Source: CAD feature listing. Evaluate the final solid. Frame: model axes, mm. A direction names the side the tool comes from. Round coordinates to 2 decimals unless told otherwise and drop trailing zeros. Write each loop counter-clockwise with the first axis right and the second up, starting at its lowest first coordinate (ties: lowest second). Pieces come first, ordered by that corner, then holes.
```python
from build123d import *

# Parameters (mm, degrees)
BOSS_EXTRUDE1_DEPTH = 3
SKETCH2_R           = 2.1
CUT_EXTRUDE1_DEPTH  = 3
BOSS_EXTRUDE2_DEPTH = 27
CUT_EXTRUDE2_DEPTH  = 27
RIB1_REACH          = 75.171
SKETCH5_WALL_W      = 155.413132852
SKETCH5_WALL_H      = 1
RIB2_REACH          = 75.171
SKETCH6_WALL_W      = 155.413132852
SKETCH6_WALL_H      = 1


with BuildPart() as part:
    # Sketch1 → Boss-Extrude1 (new body)
    with BuildSketch(Plane(origin=(0, 0, 0), x_dir=(1, 0, 0), z_dir=(0, 1, 0))):
        Polygon((0, 0), (0, 23), (12, 23), (12, 3), (52, 3), (52, 23), (64, 23), (64, 0), align=None)
    extrude(amount=-BOSS_EXTRUDE1_DEPTH)

    # Sketch2 → Cut-Extrude1 (cut)
    with BuildSketch(Plane(origin=(0, -3, 0), x_dir=(-1, 0, 0), z_dir=(0, -1, 0))):
        with Locations(Location((-6, 18.9, 0), (0, 0, 90))):
            Circle(SKETCH2_R)
        with Locations(Location((-6, 7.1, 0), (0, 0, 90))):
            Circle(SKETCH2_R)
        with Locations(Location((-58, 7.1, 0), (0, 0, 270))):
            Circle(SKETCH2_R)
        with Locations(Location((-58, 18.9, 0), (0, 0, 270))):
            Circle(SKETCH2_R)
    extrude(amount=-CUT_EXTRUDE1_DEPTH, mode=Mode.SUBTRACT)

    # Sketch3 → Boss-Extrude2 (add)
    with BuildSketch(Plane(origin=(0, 0, 0), x_dir=(1, 0, 0), z_dir=(0, 1, 0))):
        Polygon((52, 3), (12, 3), (0, 3), (0, 0), (64, 0), (64, 3), align=None)
    extrude(amount=BOSS_EXTRUDE2_DEPTH)

    # Sketch4 → Cut-Extrude2 (cut)
    with BuildSketch(Plane(origin=(0, 0, -3), x_dir=(-1, 0, 0), z_dir=(0, 0, -1))):
        with BuildLine():
            Line((-56.95, 23.5), (-56.95, 3.5))
            ThreePointArc((-56.95, 3.5), (-59, 1.45), (-61.05, 3.5))
            Line((-61.05, 3.5), (-61.05, 23.5))
            ThreePointArc((-61.05, 23.5), (-59, 25.55), (-56.95, 23.5))
        make_face()
        with BuildLine():
            Line((-7.05, 23.5), (-7.05, 3.5))
            ThreePointArc((-7.05, 3.5), (-5, 1.45), (-2.95, 3.5))
            Line((-2.95, 3.5), (-2.95, 23.5))
            ThreePointArc((-2.95, 23.5), (-5, 25.55), (-7.05, 23.5))
        make_face()
    extrude(amount=-CUT_EXTRUDE2_DEPTH, mode=Mode.SUBTRACT)

    # Sketch5 wall → Rib1 (add, up to next)
    with BuildSketch(Plane(origin=(64, 2.5, -5.5), x_dir=(0, -0.707106781187, -0.707106781187), z_dir=(0, 0.707106781187, -0.707106781187)), mode=Mode.PRIVATE) as rib1_sk1:
        with Locations((0, 0.5)):
            Rectangle(SKETCH5_WALL_W, SKETCH5_WALL_H)
    rib1_tool1 = extrude(rib1_sk1.sketch, amount=-RIB1_REACH, mode=Mode.PRIVATE) - part.part
    add(rib1_tool1.solids().sort_by_distance((64, 2.5, -5.5))[0])

    # Sketch6 wall → Rib2 (add, up to next)
    with BuildSketch(Plane(origin=(0, 2.5, -5.5), x_dir=(0, -0.707106781187, -0.707106781187), z_dir=(0, 0.707106781187, -0.707106781187)), mode=Mode.PRIVATE) as rib2_sk1:
        with Locations((0, -0.5)):
            Rectangle(SKETCH6_WALL_W, SKETCH6_WALL_H)
    rib2_tool1 = extrude(rib2_sk1.sketch, amount=-RIB2_REACH, mode=Mode.PRIVATE) - part.part
    add(rib2_tool1.solids().sort_by_distance((0, 2.5, -5.5))[0])


solid = part.part
```
Q1. Section query C-C, the plane z = -7.1. Output: boundary loops of the cut face in (x, y).
Q2. Section query B-B, the plane y = 13.5. Output: boundary loops of the cut face in (x, z), and give its area (3 significant figures).
Q3. Mould query, pull axis Z, two halves, no side actions, for faces 6 (the face through (63.5, 2.5, -5.5)), 7 (the face through (6.631, -1.521, -20.903)), 8 (the face through (61.05, 13, -2)). Classes: pulls with the +Z half, pulls with the -Z half, needs draft (parallel to the pull), parting line crosses it, or undercut.
Q4. Pin query (flat end, axial travel): P1, Ø9.5, axis at x = 8, z = -10, coming from the +Y side; P2, Ø9, axis at x = 40, y = 9.5, coming from the -Z side. Return the tip coordinate at first contact, or that it passes through.
Q5. Line query: line 1 (X direction, y = -0.8, z = -7.1); line 2 (X direction, y = 18.5, z = -2); line 3 (X direction, y = -1.5, z = -4.25). Output: solid intervals per line, ascending.
Q6. Section query D-D, the plane x = 58. Output: boundary loops of the cut face in (y, z).
Q7. Section query A-A, the plane z = -11.5. Output: boundary loops of the cut face in (x, y).
Q8. Set-up query: faces 1 (the face through (32, -3, -1)), 2 (the face through (64, 4, -3)), 3 (the face through (12, -1, -13)), 4 (the face through (63, 2, -5)), 5 (the face through (56.95, 14, -2)). Return all of +Z, -Z, +X, -X, +Y, -Y with unobstructed straight access to the full face (end or side cutting, diameter ignored); none if empty.
Filled in:
1. outline: (0, -3) - (3.9, -3) - (3.9, 0) - (1, 0) - (1, 0.9) - (0, 0.9) - close; (8.1, -3) - (12, -3) - (12, 0) - (8.1, 0) - close; (52, -3) - (55.9, -3) - (55.9, 0) - (52, 0) - close; (60.1, -3) - (64, -3) - (64, 0.9) - (63, 0.9) - (63, 0) - (60.1, 0) - close
2. outline: (0, -3) - (2.95, -3) - (2.95, 0) - (0, 0) - close; (7.05, -3) - (56.95, -3) - (56.95, 0) - (7.05, 0) - close; (61.05, -3) - (64, -3) - (64, 0) - (61.05, 0) - close
2. area: 167 mm2
3. face 6: pulls with the -Z half
3. face 7: undercut
3. face 8: needs draft
4. P1: stops at y = 0
4. P2: stops at z = -3
5. line 1: x = 0 to 3.9, 8.1 to 12, 52 to 55.9, 60.1 to 64
5. line 2: x = 0 to 2.95, 7.05 to 56.95, 61.05 to 64
5. line 3: x = 0 to 12, 52 to 64
6. outline: (-3, -23) - (0, -23) - (0, -21) - (-3, -21) - close; (-3, -16.8) - (0, -16.8) - (0, -9.2) - (-3, -9.2) - close; (-3, -5) - (0, -5) - (0, -3) - (1.71, -3) - (1.71, 0) - (-3, 0) - close; (25.29, -3) - (27, -3) - (27, 0) - (25.29, 0) - close
7. outline: (0, -3) - (12, -3) - (12, 0) - (0, 0) - close; (52, -3) - (64, -3) - (64, 0) - (52, 0) - close
8. face 1: +Z, -Z, +X, -X, -Y
8. face 2: +Z, -Z, +X, +Y, -Y
8. face 3: -Z, +Y, -Y
8. face 4: -Z, +Y
8. face 5: +Z, -Z
